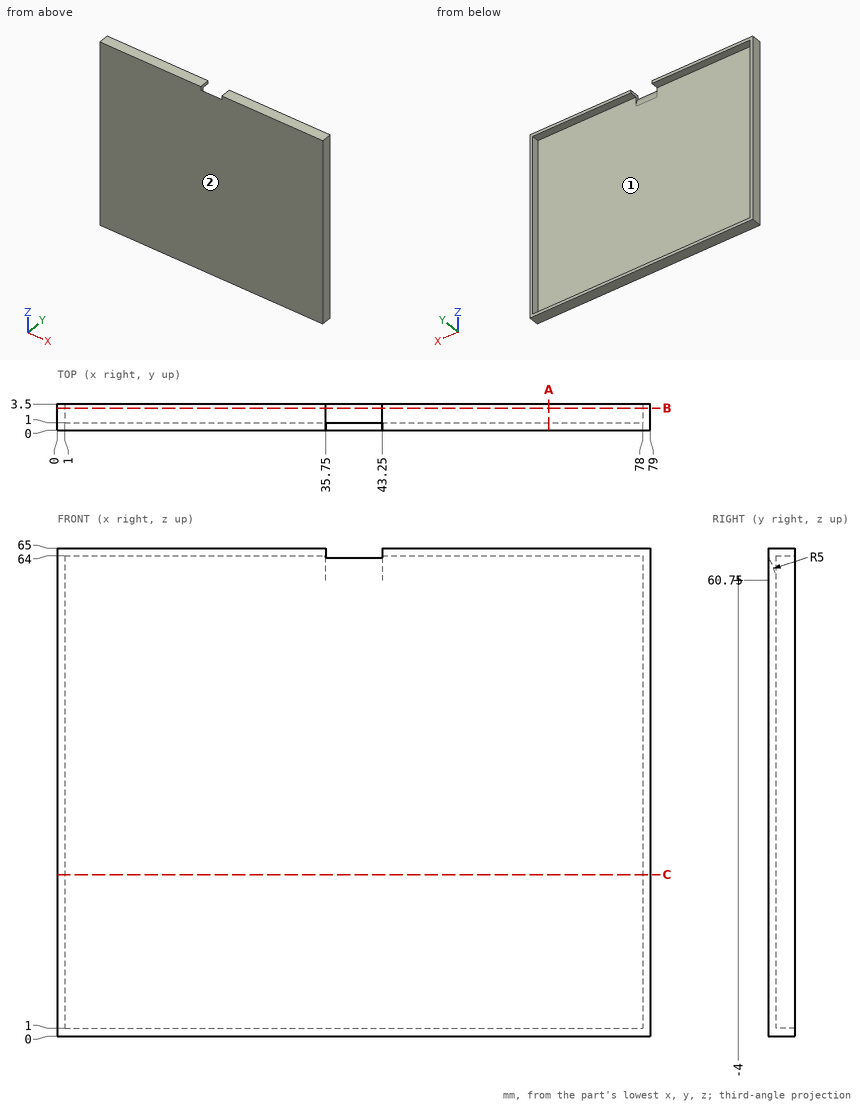
Design review of the part shown in the three views and the two pictorial views. Dimensions are in mm from the part's minimum x, y and z. Round coordinates to 2 decimals unless told otherwise and drop trailing zeros. Loops run counter-clockwise (first coordinate to the right, second up) from the corner with the lowest first, then second, coordinate; pieces in that order, holes last. Notation, with made-up numbers: (8.5, 52.5) - (59.5, 52.5) arc R19 ccw to (59.5, 79.5) - close; hole circle Ø2 at (-13.75, -9). An arc over 180 degrees is marked (long way). One line per item, written item: value. Start each with the question number.
Item 1: Clearance check with flat-ended pins moving along their axes: pin 1 Ø0.8 at (y, z) = (2, 28) entering from -X; pin 2 Ø6 at (x, z) = (22, 49) entering from +Y. State where each tip first meets the part, or that it passes through.
Item 2: For L1, parallel to X at y = 2.7, z = 31; L2, parallel to Z at x = 62.5, y = 1.4; L3, parallel to Y at x = 4.5, z = 25, list the stretches that pass through material, from the lowest coordinate up.
Item 3: Take a section at B-B (y = 2.95). Give the boundary of the cut face in (x, z).
Item 4: Take a section at A-A (x = 65.5). Give the boundary of the cut face in (y, z), plus the area to 3 significant figures.
Item 5: Take a section at C-C (z = 21.5). Give the boundary of the cut face in (x, y), plus the area to 3 significant figures.
Item 6: The part is to be moulded in two halves that separate along X. For the marked faces 1 and 2, say which applies: +X half, -X half, draft (parallel to the pull), parting line (faces both ways), or undercut.
Answer below:
1. pin 1: stops at x = 0
1. pin 2: stops at y = 1
2. L1: x = 0 to 1, 78 to 79
2. L2: z = 0 to 1, 64 to 65
2. L3: y = 0 to 1
3. outline: (0, 0) - (79, 0) - (79, 65) - (43.25, 65) - (43.25, 64) - (78, 64) - (78, 1) - (1, 1) - (1, 64) - (35.75, 64) - (35.75, 65) - (0, 65) - close
4. outline: (0, 0) - (3.5, 0) - (3.5, 1) - (1, 1) - (1, 64) - (3.5, 64) - (3.5, 65) - (0, 65) - close
4. area: 70.0 mm2
5. outline: (0, 0) - (79, 0) - (79, 3.5) - (78, 3.5) - (78, 1) - (1, 1) - (1, 3.5) - (0, 3.5) - close
5. area: 84.0 mm2
6. face 1: undercut
6. face 2: draft
